```python
from build123d import *

# Parameters (mm, degrees)
SKETCH_1_R          = 1.8
EXTRUDE_1_DEPTH     = 6
CUT_EXTRUDE_1_DEPTH = 3
FILLET_1_R          = 2


with BuildPart() as part:
    # ｽｹｯﾁ1 → ﾎﾞｽ - 押し出し1 (new body)
    with BuildSketch(Plane.XY):
        with BuildLine():
            Line((-68.800816256, 45.189746609), (-2.800816256, 45.189746609))
            ThreePointArc((-2.800816256, 45.189746609), (0.73471765, 43.725280515), (2.199183744, 40.189746609))
            Line((2.199183744, 40.189746609), (-1.800816256, 21.189746609))
            ThreePointArc((-1.800816256, 21.189746609), (-5.800816256, 17.944170221), (-9.800816256, 21.189746609))
            Line((-9.800816256, 21.189746609), (-11.537510812, 27.036945787))
            ThreePointArc((-11.537510812, 27.036945787), (-15.143316964, 32.20448278), (-21.123618303, 34.189746609))
            Line((-21.123618303, 34.189746609), (-50.478014208, 34.189746609))
            ThreePointArc((-50.478014208, 34.189746609), (-56.458315547, 32.20448278), (-60.0641217, 27.036945787))
            Line((-60.0641217, 27.036945787), (-61.800816256, 21.189746609))
            ThreePointArc((-61.800816256, 21.189746609), (-65.800816256, 17.944170221), (-69.800816256, 21.189746609))
            Line((-69.800816256, 21.189746609), (-73.800816256, 40.189746609))
            ThreePointArc((-73.800816256, 40.189746609), (-72.336350162, 43.725280515), (-68.800816256, 45.189746609))
        make_face()
        with Locations((-68.800816256, 40.189746609)):
            Circle(SKETCH_1_R, mode=Mode.SUBTRACT)
        with Locations((-65.800816256, 21.189746609)):
            Circle(SKETCH_1_R, mode=Mode.SUBTRACT)
        with Locations((-5.800816256, 21.189746609)):
            Circle(SKETCH_1_R, mode=Mode.SUBTRACT)
        with Locations((-2.800816256, 40.189746609)):
            Circle(SKETCH_1_R, mode=Mode.SUBTRACT)
    extrude(amount=EXTRUDE_1_DEPTH)

    # ｽｹｯﾁ2 → ｶｯﾄ - 押し出し1 (cut)
    with BuildSketch(Plane.XY.offset(6)):
        Polygon((-60.0641217, 27.036945787), (-11.537510812, 27.036945787), (-7.715868533, 45.189746609), (-63.885763978, 45.189746609), align=None)
    extrude(amount=-CUT_EXTRUDE_1_DEPTH, mode=Mode.SUBTRACT)

    # ﾌｨﾚｯﾄ1
    fillet_1_edges = [part.edges().sort_by_distance(p)[0] for p in [
        (-11.537510812, 27.036945787, 4.5),
        (-60.0641217, 27.036945787, 4.5),
        (-63.885763978, 45.189746609, 4.5),
        (-7.715868533, 45.189746609, 4.5),
    ]]
    fillet(fillet_1_edges, radius=FILLET_1_R)


solid = part.part
```
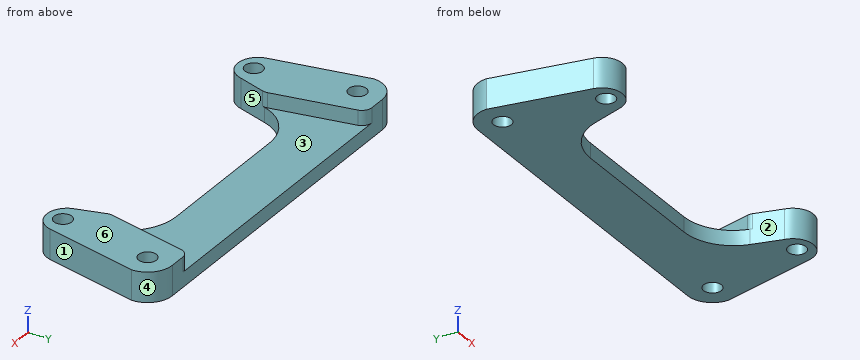
Build history of the part. All positions in model axes, mm. Face numbers are marked on the shaded views. A direction names the side the tool comes from. Coordinates: 2 decimals unless noted, no trailing zeros. Order: outer loops, then holes, each group sorted by start corner. A loop starts at its lowest first (then second) coordinate and runs counter-clockwise, first axis right, second up. Notation, with made-up numbers: M -3.5,18.25 L 52.5,18.25 A26 ccw 52.5,57.25 Z; hole C -10.75,-35 d9. An arc over 180 degrees is marked long. One line per question, with ' | ' between items. Start each with the question number.
1. Cut at D-D (x = -9). Write the cut outline in (y, z).
2. Cut at B-B (z = 1.3). Write the cut outline in (x, y), plus the area to 3 significant figures.
3. Mould opens along X. For the marked faces 3, 4, 5 and 6 say: +X half, -X half, draft (parallel to the pull), parting line (faces both ways), or undercut.
4. Flat gauge pins, fed straight in: P1, Ø1, axis at x = -15.5, z = 4, coming from the +Y side; P2, Ø9.5, axis at x = -37.5, y = 36.5, coming from the +Z side; P3, Ø2.5, axis at x = -41, z = 1.5, coming from the -Y side. Where does each tip first touch, or does it go through?
5. Cut at C-C (y = 41). Write the cut outline in (x, z).
6. Tool access for the marked faces 1 and 2: list every direction of +Z, -Z, +X, -X, +Y, -Y with a clear straight run to the whole face (end or side of a thin tool).
7. Wall check: line 1 along Y through (x, z) = (-6, 2.45); line 2 along X through (y, z) = (39, 0.8); line 3 along Y through (x, z) = (-23.5, 0.5). Give the ranges that are in metal, low to high. Write a range as [from, to].
8. Cut at A-A (z = 4.3). Write the cut outline in (x, y), plus the area to 3 significant figures.
The answers:
1) outline: M 19.49,0 L 45.19,0 L 45.19,3 L 39.09,3 L 39.09,6 L 19.49,6 Z
2) outline: M -73.8,40.19 L -69.8,21.19 A4.09 ccw -61.8,21.19 L -60.06,27.04 A10 cw -50.48,34.19 L -21.12,34.19 A10 cw -11.54,27.04 L -9.8,21.19 A4.09 ccw -1.8,21.19 L 2.2,40.19 A5 ccw -2.8,45.19 L -68.8,45.19 A5 ccw Z; hole C -68.8,40.19 d3.6; hole C -65.8,21.19 d3.6; hole C -5.8,21.19 d3.6; hole C -2.8,40.19 d3.6 | area: 1,130 mm2
3) face 3: undercut | face 4: +X half | face 5: undercut | face 6: draft
4) P1: passes through | P2: stops at z = 3 | P3: stops at y = 34.19
5) outline: M -73.73,0 L -70.41,0 L -70.41,6 L -73.73,6 Z; M -67.19,0 L -4.41,0 L -4.41,6 L -8.6,6 L -8.6,3 L -63,3 L -63,6 L -67.19,6 Z; M -1.19,0 L 2.13,0 L 2.13,6 L -1.19,6 Z
6) face 1: +Z, -Z, +X, -Y | face 2: +Z, -Z, -Y
7) line 1: y = [17.95, 19.4], [22.98, 45.19] | line 2: x = [-73.55, -70.15], [-67.45, -4.15], [-1.45, 1.95] | line 3: y = [34.19, 45.19]
8) outline: M -73.8,40.19 L -69.8,21.19 A4.09 ccw -61.8,21.19 L -60.21,26.55 A2 ccw -60.17,27.53 L -63.55,43.6 A2 ccw -65.51,45.19 L -68.8,45.19 A5 ccw Z; M -11.43,27.53 A2 ccw -11.39,26.55 L -9.8,21.19 A4.09 ccw -1.8,21.19 L 2.2,40.19 A5 ccw -2.8,45.19 L -6.09,45.19 A2 ccw -8.05,43.6 Z; hole C -68.8,40.19 d3.6; hole C -65.8,21.19 d3.6; hole C -5.8,21.19 d3.6; hole C -2.8,40.19 d3.6 | area: 490 mm2
